Build history of the part. All positions in model axes, mm. A direction names the side the tool comes from. Give positions to 0.01 mm unless a question says otherwise; leave off trailing zeros. Order: outer loops, then holes, each group sorted by start corner. A loop starts at its lowest first (then second) coordinate and runs counter-clockwise, first axis right, second up. Notation, with made-up numbers: (23.5, 52.25) -> (27.5, 52.25) arc R14 cw to (27.5, 61.25) -> close; hole circle Ø1 at (12, -21). An arc over 180 degrees is marked (long way). Use a Markdown table: item, result. Add a question column.
```python
from build123d import *

# Parameters (mm, degrees)
SKETCH1_W                = 31.75
SKETCH1_H                = 12.7
BOSS_EXTRUDE1_DEPTH      = 6.35
SKETCH3_W                = 25.4
SKETCH3_H                = 5.08
CUT_EXTRUDE1_DEPTH       = 2.54
BOSS_EXTRUDE2_DEPTH      = 3.81
SKETCH5_W                = 31.75
SKETCH5_H                = 6.35
BOSS_EXTRUDE3_DEPTH      = 8.89
SKETCH6_W                = 25.4
SKETCH6_H                = 5.08
CUT_EXTRUDE2_DEPTH       = 2.54
SKETCH9_W                = 6.35
SKETCH9_H                = 3.81
BOSS_EXTRUDE5_DEPTH      = 6.35
SKETCH10_W               = 6.35
SKETCH10_H               = 6.35
BOSS_EXTRUDE6_DEPTH      = 12.9159
SKETCH12_W               = 6.35
SKETCH12_H               = 3.81
BOSS_EXTRUDE8_DEPTH      = 6.35
SKETCH14_W               = 6.35
SKETCH14_H               = 6.35
BOSS_EXTRUDE11_DEPTH     = 19.05
CUT_EXTRUDE9_DEPTH       = 101.12747092
SKETCH19_W               = 72.39
SKETCH19_H               = 3.81
BOSS_EXTRUDE12_DEPTH     = 34.163
BOSS_EXTRUDE13_DEPTH     = 27.813
SKETCH21_W               = 12.7
SKETCH21_H               = 3.81
CUT_EXTRUDE10_DEPTH      = 7.62
SKETCH22_W               = 41.91
SKETCH22_H               = 3.81
BOSS_EXTRUDE14_DEPTH     = 50.8
SKETCH23_W               = 85.09
SKETCH23_H               = 3.81
BOSS_EXTRUDE15_DEPTH     = 44.45
SKETCH24_R               = 1.5
CUT_EXTRUDE11_DEPTH      = 149.400241239
SKETCH25_W               = 41.91
SKETCH25_H               = 3.81
BOSS_EXTRUDE16_DEPTH     = 6.35
CUT_EXTRUDE12_DEPTH      = 154.181474728
CUT_EXTRUDE12_DEPTH_BACK = 154.181474728
CUT_EXTRUDE13_DEPTH      = 1.27
CHAMFER1_SIZE            = 6.35
CHAMFER1_SIZE_2          = 2.565566534


with BuildPart() as part:
    # Sketch1 → Boss-Extrude1 (new body)
    with BuildSketch(Plane.XY):
        with Locations((15.875, 6.35)):
            Rectangle(SKETCH1_W, SKETCH1_H)
    extrude(amount=BOSS_EXTRUDE1_DEPTH)

    # Sketch3 → Cut-Extrude1 (cut)
    with BuildSketch(Plane.XY.offset(6.35)):
        with Locations((12.7, 6.35)):
            Rectangle(SKETCH3_W, SKETCH3_H)
    extrude(amount=-CUT_EXTRUDE1_DEPTH, mode=Mode.SUBTRACT)

    # Sketch4 → Boss-Extrude2 (add)
    with BuildSketch(Plane(origin=(0, 12.7, 0), x_dir=(1, 0, 0), z_dir=(0, 1, 0))):
        Polygon((0, 0), (-25.4, 0), (-25.4, -97.79), (31.75, -97.79), (31.75, -91.44), (-19.05, -91.44), (-19.05, -6.35), (0, -6.35), align=None)
    extrude(amount=-BOSS_EXTRUDE2_DEPTH)

    # Sketch5 → Boss-Extrude3 (add)
    with BuildSketch(Plane.XZ.offset(-8.89)):
        with Locations((15.875, 94.615)):
            Rectangle(SKETCH5_W, SKETCH5_H)
    extrude(amount=BOSS_EXTRUDE3_DEPTH)

    # Sketch6 → Cut-Extrude2 (cut)
    with BuildSketch(Plane(origin=(0, 0, 91.44), x_dir=(-1, 0, 0), z_dir=(0, 0, -1))):
        with Locations((-12.7, 6.35)):
            Rectangle(SKETCH6_W, SKETCH6_H)
    extrude(amount=-CUT_EXTRUDE2_DEPTH, mode=Mode.SUBTRACT)

    # Sketch9 → Boss-Extrude5 (add)
    with BuildSketch(Plane.ZY.offset(25.4)):
        with Locations((88.265, 10.795)):
            Rectangle(SKETCH9_W, SKETCH9_H)
        with Locations((9.525, 10.795)):
            Rectangle(SKETCH9_W, SKETCH9_H)
    extrude(amount=BOSS_EXTRUDE5_DEPTH)

    # Sketch10 → Boss-Extrude6 (add)
    with BuildSketch(Plane(origin=(0, 12.7, 0), x_dir=(1, 0, 0), z_dir=(0, 1, 0))):
        with Locations((-28.575, -88.265)):
            Rectangle(SKETCH10_W, SKETCH10_H)
        with Locations((-28.575, -9.525)):
            Rectangle(SKETCH10_W, SKETCH10_H)
    extrude(amount=BOSS_EXTRUDE6_DEPTH)

    # Sketch12 → Boss-Extrude8 (add)
    with BuildSketch(Plane.ZY.offset(25.4)):
        with Locations((94.615, 10.795)):
            Rectangle(SKETCH12_W, SKETCH12_H)
        with Locations((3.175, 10.795)):
            Rectangle(SKETCH12_W, SKETCH12_H)
    extrude(amount=BOSS_EXTRUDE8_DEPTH)

    # Sketch14 → Boss-Extrude11 (add)
    with BuildSketch(Plane(origin=(-25.4, 0, 0), x_dir=(0, 0, -1), z_dir=(1, 0, 0))):
        with Locations((-88.265, 22.4409)):
            Rectangle(SKETCH14_W, SKETCH14_H)
        with Locations((-9.525, 22.4409)):
            Rectangle(SKETCH14_W, SKETCH14_H)
    extrude(amount=BOSS_EXTRUDE11_DEPTH)

    # Sketch18 → Cut-Extrude9 (cut, through all)
    with BuildSketch(Plane.XY.offset(91.44)):
        Polygon((-31.75, 19.15795), (-25.4, 25.6159), (-31.75, 25.6159), align=None)
    extrude(amount=-CUT_EXTRUDE9_DEPTH, mode=Mode.SUBTRACT)

    # Sketch19 → Boss-Extrude12 (add)
    with BuildSketch(Plane.ZY.offset(25.4)):
        with Locations((48.895, 10.795)):
            Rectangle(SKETCH19_W, SKETCH19_H)
    extrude(amount=BOSS_EXTRUDE12_DEPTH)

    # Sketch20 → Boss-Extrude13 (add)
    with BuildSketch(Plane.ZY.offset(31.75)):
        Polygon((0, 8.89), (0, 12.7), (6.35, 12.7), (6.35, 19.15795), (12.7, 19.15795), (12.7, 8.89), align=None)
        Polygon((85.09, 19.15795), (91.44, 19.15795), (91.44, 12.7), (97.79, 12.7), (97.79, 8.89), (85.09, 8.89), align=None)
    extrude(amount=BOSS_EXTRUDE13_DEPTH)

    # Sketch21 → Cut-Extrude10 (cut)
    with BuildSketch(Plane.ZY.offset(59.563)):
        with Locations((21.59, 10.795)):
            Rectangle(SKETCH21_W, SKETCH21_H)
        with Locations((76.2, 10.795)):
            Rectangle(SKETCH21_W, SKETCH21_H)
    extrude(amount=-CUT_EXTRUDE10_DEPTH, mode=Mode.SUBTRACT)

    # Sketch22 → Boss-Extrude14 (add)
    with BuildSketch(Plane.ZY.offset(59.563)):
        with Locations((48.895, 10.795)):
            Rectangle(SKETCH22_W, SKETCH22_H)
    extrude(amount=BOSS_EXTRUDE14_DEPTH)

    # Sketch23 → Boss-Extrude15 (add)
    with BuildSketch(Plane(origin=(-19.05, 0, 0), x_dir=(0, 0, -1), z_dir=(1, 0, 0))):
        with Locations((-48.895, 10.795)):
            Rectangle(SKETCH23_W, SKETCH23_H)
    extrude(amount=BOSS_EXTRUDE15_DEPTH)

    # Sketch24 → Cut-Extrude11 (cut, through all)
    with BuildSketch(Plane.XZ.offset(-8.89)):
        with Locations(Location((-107.823, 30.353, 0), (0, 0, 270))):
            Circle(SKETCH24_R)
        with Locations(Location((-107.823, 67.437, 0), (0, 0, 270))):
            Circle(SKETCH24_R)
    extrude(amount=-CUT_EXTRUDE11_DEPTH, mode=Mode.SUBTRACT)

    # Sketch25 → Boss-Extrude16 (add)
    with BuildSketch(Plane.ZY.offset(110.363)):
        with Locations((48.895, 10.795)):
            Rectangle(SKETCH25_W, SKETCH25_H)
    extrude(amount=BOSS_EXTRUDE16_DEPTH)

    # Sketch26 → Cut-Extrude12 (cut, two sides: drawn at the far end of the back side and taken through both)
    with BuildSketch(Plane.XZ.offset(-8.89).offset(-CUT_EXTRUDE12_DEPTH_BACK)):
        Polygon((25.4, 37.973), (25.4, 48.895), (25.4, 59.817), (5.08, 59.817), (5.08, 37.973), align=None)
    extrude(amount=CUT_EXTRUDE12_DEPTH + CUT_EXTRUDE12_DEPTH_BACK, mode=Mode.SUBTRACT)

    # Sketch27 → Cut-Extrude13 (cut)
    with BuildSketch(Plane.XZ.offset(-8.89)):
        Polygon((25.4, 37.973), (25.4, 6.35), (-38.1, 6.35), (-38.1, 91.44), (25.4, 91.44), (25.4, 59.817), (5.08, 59.817), (5.08, 37.973), align=None)
    extrude(amount=-CUT_EXTRUDE13_DEPTH, mode=Mode.SUBTRACT)

    # Chamfer1
    # the kernel refuses this chamfer: 6.35, 2.565566534 mm, written as the material it takes off along each edge
    with BuildSketch(Plane(origin=(5.08, 12.7, 59.817), x_dir=(0, 0.014446902557764131, 0.9998956380575357), z_dir=(1, 0, 0)), Plane(origin=(41.865480117, 12.7, 37.973), x_dir=(0, 0.014446902557764124, -0.9998956380575357), z_dir=(-1, 0, 0))) as chamfer1_piece_1:
        Polygon((CHAMFER1_SIZE * 0.999895638058, CHAMFER1_SIZE * 0.0144469025578), (-CHAMFER1_SIZE_2 * 0.0144469025581, CHAMFER1_SIZE_2 * 0.999895638078), (0, 0), align=None)
    extrude(amount=36.785480117, mode=Mode.SUBTRACT)
    with BuildSketch(Plane(origin=(5.08, 12.7, 37.973), x_dir=(-0.9998956380575357, 0.01444690255776412, 0), z_dir=(0, 0, 1))) as chamfer1_piece_2:
        Polygon((CHAMFER1_SIZE * 0.999895638058, CHAMFER1_SIZE * 0.0144469025578), (-CHAMFER1_SIZE_2 * 0.0144469025581, CHAMFER1_SIZE_2 * 0.999895638078), (0, 0), align=None)
    extrude(amount=21.844, mode=Mode.SUBTRACT)
    with BuildSketch(Plane(origin=(-11.385480117, 12.7, 59.817), x_dir=(0, 0.014446902557764131, 0.9998956380575357), z_dir=(1, 0, 0))) as chamfer1_piece_3a_section:
        Polygon((CHAMFER1_SIZE * 0.999895638058, CHAMFER1_SIZE * 0.0144469025578), (-CHAMFER1_SIZE_2 * 0.0144469025581, CHAMFER1_SIZE_2 * 0.999895638078), (0, 0), align=None)
    chamfer1_piece_3a = extrude(amount=53.250960234, mode=Mode.PRIVATE)
    chamfer1_piece_3a = split(chamfer1_piece_3a, bisect_by=Plane(origin=(5.08, 11.901985968, 61.978678206), z_dir=(-1, 0, 0)), keep=Keep.TOP, mode=Mode.PRIVATE)
    with BuildSketch(Plane(origin=(5.08, 12.7, 37.973), x_dir=(-0.9998956380575357, 0.01444690255776412, 0), z_dir=(0, 0, 1))) as chamfer1_piece_3b_section:
        Polygon((CHAMFER1_SIZE * 0.999895638058, CHAMFER1_SIZE * 0.0144469025578), (-CHAMFER1_SIZE_2 * 0.0144469025581, CHAMFER1_SIZE_2 * 0.999895638078), (0, 0), align=None)
    chamfer1_piece_3b = extrude(amount=38.309480117, mode=Mode.PRIVATE)
    chamfer1_piece_3b = split(chamfer1_piece_3b, bisect_by=Plane(origin=(2.918321794, 11.901985968, 59.817), z_dir=(0, 0, 1)), keep=Keep.TOP, mode=Mode.PRIVATE)
    chamfer1_piece_3 = chamfer1_piece_3a & chamfer1_piece_3b
    add(chamfer1_piece_3, mode=Mode.SUBTRACT)
    with BuildSketch(Plane(origin=(5.08, 12.7, 21.507519883), x_dir=(-0.9998956380575357, 0.01444690255776412, 0), z_dir=(0, 0, 1))) as chamfer1_piece_4a_section:
        Polygon((CHAMFER1_SIZE * 0.999895638058, CHAMFER1_SIZE * 0.0144469025578), (-CHAMFER1_SIZE_2 * 0.0144469025581, CHAMFER1_SIZE_2 * 0.999895638078), (0, 0), align=None)
    chamfer1_piece_4a = extrude(amount=38.309480117, mode=Mode.PRIVATE)
    chamfer1_piece_4a = split(chamfer1_piece_4a, bisect_by=Plane(origin=(2.918321794, 11.901985968, 37.973), z_dir=(0, 0, -1)), keep=Keep.TOP, mode=Mode.PRIVATE)
    with BuildSketch(Plane(origin=(41.865480117, 12.7, 37.973), x_dir=(0, 0.014446902557764124, -0.9998956380575357), z_dir=(-1, 0, 0))) as chamfer1_piece_4b_section:
        Polygon((CHAMFER1_SIZE * 0.999895638058, CHAMFER1_SIZE * 0.0144469025578), (-CHAMFER1_SIZE_2 * 0.0144469025581, CHAMFER1_SIZE_2 * 0.999895638078), (0, 0), align=None)
    chamfer1_piece_4b = extrude(amount=53.250960234, mode=Mode.PRIVATE)
    chamfer1_piece_4b = split(chamfer1_piece_4b, bisect_by=Plane(origin=(5.08, 11.901985968, 35.811321794), z_dir=(-1, 0, 0)), keep=Keep.TOP, mode=Mode.PRIVATE)
    chamfer1_piece_4 = chamfer1_piece_4a & chamfer1_piece_4b
    add(chamfer1_piece_4, mode=Mode.SUBTRACT)


solid = part.part
```
(1) Mould opens along Z. For faces 1 (the face through (31.75, 6, 3)), 2 (the face through (-33, 18, 91.44)), 3 (the face through (-108.74, 10.77, 31.54)) say: released by +Z, released by -Z, zero draft, split by the parting line, or undercut.
(2) Band-saw the part on A-A on x = -17. Give the cut face in (y, z).
(3) Tool access for faces 4 (the face through (-33, 18, 85.09)), 5 (the face through (1.829, 11.448, 48.653)), 6 (the face through (-56, 11, 82.55)), 7 (the face through (-6.35, 22, 10)): list every direction of +Z, -Z, +X, -X, +Y, -Y with a clear straight run to the whole face (end or side of a thin tool).
(4) Pin check, flat tips, straight feed: pin 1 Ø3 at (y, z) = (15, 8.5) entering from +X; pin 2 Ø1 at (x, z) = (-66.5, 65.5) entering from -Y; pin 3 Ø10 at (x, y) = (-70.5, 14.5) entering from -Z. Stop position of each tip, or through.
(5) Band-saw the part on D-D on x = -40.5. Give the cut face in (y, z), plus the area to 3 significant figures.
(6) Band-saw the part on B-B on y = 6.25. Give the cut face in (x, z).
(7) Wall check: probe 1 along Z at (x, y) = (-108, 10.5); probe 2 along Z at (x, y) = (-51.5, 14.5); probe 3 along Y at (x, z) = (-39.5, 18). Give the ranges that are in metal, low to high.
(8) Band-saw the part on C-C on z = 88.5. Give the cut face in (x, y).
Response:
| question | item | result |
|---|---|---|
| 1 | face 1 | zero draft |
| 1 | face 2 | released by +Z |
| 1 | face 3 | undercut |
| 2 | outline | (8.89, 0) -> (12.7, 0) -> (12.7, 97.79) -> (8.89, 97.79) -> (8.89, 91.44) -> (10.16, 91.44) -> (10.16, 6.35) -> (8.89, 6.35) -> close; (19.27, 6.35) -> (25.62, 6.35) -> (25.62, 12.7) -> (19.27, 12.7) -> close; (19.27, 85.09) -> (25.62, 85.09) -> (25.62, 91.44) -> (19.27, 91.44) -> close |
| 3 | face 4 | +X, -X, +Y |
| 3 | face 5 | +X, +Y |
| 3 | face 6 | -X, +Y, -Y |
| 3 | face 7 | +Z, -Z, +X, +Y |
| 4 | pin 1 | stops at x = -25.4 |
| 4 | pin 2 | stops at y = 8.89 |
| 4 | pin 3 | stops at z = 27.94 |
| 5 | outline | (8.89, 0) -> (12.7, 0) -> (12.7, 6.35) -> (19.16, 6.35) -> (19.16, 12.7) -> (12.7, 12.7) -> (12.7, 85.09) -> (19.16, 85.09) -> (19.16, 91.44) -> (12.7, 91.44) -> (12.7, 97.79) -> (8.89, 97.79) -> close |
| 5 | area | 455 mm² |
| 6 | outline | (0, 0) -> (31.75, 0) -> (31.75, 6.35) -> (25.4, 6.35) -> (25.4, 3.81) -> (0, 3.81) -> close; (0, 93.98) -> (25.4, 93.98) -> (25.4, 91.44) -> (31.75, 91.44) -> (31.75, 97.79) -> (0, 97.79) -> close |
| 7 | probe 1 | z = 27.94 to 28.86, 31.84 to 65.95, 68.93 to 69.85 |
| 7 | probe 2 | z = 6.35 to 12.7, 85.09 to 91.44 |
| 7 | probe 3 | y = 8.89 to 12.7 |
| 8 | outline | (-59.56, 8.89) -> (-38.1, 8.89) -> (-38.1, 10.16) -> (25.4, 10.16) -> (25.4, 12.7) -> (-25.4, 12.7) -> (-25.4, 19.27) -> (-6.35, 19.27) -> (-6.35, 25.62) -> (-25.4, 25.62) -> (-31.75, 19.16) -> (-59.56, 19.16) -> close |
